Geometry: final body of the model. Coordinates: model frame, mm. A direction names the side the tool comes from. Give positions to 0.01 mm unless a question says otherwise; leave off trailing zeros. Order: outer loops, then holes, each group sorted by start corner. A loop starts at its lowest first (then second) coordinate and runs counter-clockwise, first axis right, second up. Notation, with made-up numbers: (-8.75, 43.5) - (40.25, 43.5) arc R6 ccw to (40.25, 47.5) - close; hole circle Ø11 at (-13.5, -34.5). An arc over 180 degrees is marked (long way). Use one line per item in the form item = value.
from build123d import *

# Parameters (mm, degrees)
EXTRUDE_1_DEPTH     = 20
SKETCH_2_R          = 3
CUT_EXTRUDE_1_DEPTH = 42.952353927
SKETCH_3_R          = 3
CUT_EXTRUDE_2_DEPTH = 42.952353927
SKETCH_4_W          = 2
SKETCH_4_H          = 6
EXTRUDE_1_2_DEPTH   = 1.5
SKETCH_5_W          = 4
SKETCH_5_H          = 6
CUT_EXTRUDE_3_DEPTH = 1.5
SKETCH_6_W          = 6
SKETCH_6_H          = 2
EXTRUDE_2_DEPTH     = 1.5
SKETCH_7_W          = 6
SKETCH_7_H          = 4
CUT_EXTRUDE_4_DEPTH = 1.5
SKETCH_8_W          = 6
SKETCH_8_H          = 2
EXTRUDE_3_DEPTH     = 1.5
SKETCH_10_W         = 6
SKETCH_10_H         = 2
CUT_EXTRUDE_6_DEPTH = 1.5
SKETCH_11_W         = 2
SKETCH_11_H         = 6
EXTRUDE_4_DEPTH     = 1.5
SKETCH_12_W         = 2
SKETCH_12_H         = 6
CUT_EXTRUDE_7_DEPTH = 1.5
RIB_1_DEPTH         = 2.6
RIB_START           = -2.6
RIB_2_DEPTH         = 2.6


# Read off the part's stored shape, not the designer's step: 筋1, 筋2
with BuildPart() as part:
    # 草图1 → Extrude 1 (new body)
    with BuildSketch(Plane.XY):
        Polygon((28, 0), (0, 0), (0, 28), (4, 28), (4, 4), (28, 4), align=None)
    extrude(amount=EXTRUDE_1_DEPTH)

    # 草图2 → 切除-拉伸1 (cut, through all)
    with BuildSketch(Plane(origin=(0, 4, 0), x_dir=(1, 0, 0), z_dir=(0, 1, 0))):
        with Locations(Location((17, -10, 0), (0, 0, 180))):
            Circle(SKETCH_2_R)
    extrude(amount=-CUT_EXTRUDE_1_DEPTH, mode=Mode.SUBTRACT)

    # 草图3 → 切除-拉伸2 (cut, through all)
    with BuildSketch(Plane(origin=(4, 0, 0), x_dir=(0, 0, -1), z_dir=(1, 0, 0))):
        with Locations((-10, 17)):
            Circle(SKETCH_3_R)
    extrude(amount=-CUT_EXTRUDE_2_DEPTH, mode=Mode.SUBTRACT)

    # 草图4 → Extrude 1 2 (add)
    with BuildSketch(Plane.XZ):
        with Locations((3, 10)):
            Rectangle(SKETCH_4_W, SKETCH_4_H)
    extrude(amount=EXTRUDE_1_2_DEPTH)

    # 草图5 → 切除-拉伸3 (cut)
    with BuildSketch(Plane.XZ):
        with Locations((6, 10)):
            Rectangle(SKETCH_5_W, SKETCH_5_H)
    extrude(amount=-CUT_EXTRUDE_3_DEPTH, mode=Mode.SUBTRACT)

    # 草图6 → 凸台-拉伸2 (add)
    with BuildSketch(Plane.ZY):
        with Locations((10, 3)):
            Rectangle(SKETCH_6_W, SKETCH_6_H)
    extrude(amount=EXTRUDE_2_DEPTH)

    # 草图7 → 切除-拉伸4 (cut)
    with BuildSketch(Plane.ZY):
        with Locations((10, 6)):
            Rectangle(SKETCH_7_W, SKETCH_7_H)
    extrude(amount=-CUT_EXTRUDE_4_DEPTH, mode=Mode.SUBTRACT)

    # 草图8 → 凸台-拉伸3 (add)
    with BuildSketch(Plane.ZY):
        with Locations((10, 25)):
            Rectangle(SKETCH_8_W, SKETCH_8_H)
    extrude(amount=EXTRUDE_3_DEPTH)

    # 草图10 → 切除-拉伸6 (cut)
    with BuildSketch(Plane.ZY):
        with Locations((10, 23)):
            Rectangle(SKETCH_10_W, SKETCH_10_H)
    extrude(amount=-CUT_EXTRUDE_6_DEPTH, mode=Mode.SUBTRACT)

    # 草图11 → 凸台-拉伸4 (add)
    with BuildSketch(Plane.XZ):
        with Locations((25, 10)):
            Rectangle(SKETCH_11_W, SKETCH_11_H)
    extrude(amount=EXTRUDE_4_DEPTH)

    # 草图12 → 切除-拉伸7 (cut)
    with BuildSketch(Plane.XZ):
        with Locations((23, 10)):
            Rectangle(SKETCH_12_W, SKETCH_12_H)
    extrude(amount=-CUT_EXTRUDE_7_DEPTH, mode=Mode.SUBTRACT)

    # 筋1 outline → 筋1 (add)
    with BuildSketch(Plane.XY):
        Polygon((6, 23), (6, 28), (4, 28), (4, 4), (28, 4), (28, 6), (23, 6), align=None)
    extrude(amount=RIB_1_DEPTH)

    # 筋2 outline → 筋2 (add)
    with BuildSketch(Plane.XY.offset(20).offset(RIB_START)):
        Polygon((6, 23), (6, 28), (4, 28), (4, 4), (28, 4), (28, 6), (23, 6), align=None)
    extrude(amount=RIB_2_DEPTH)


solid = part.part
(1) Pull-direction query (X, two-part tool) for faces 1 (the face through (26, -1, 10)), 2 (the face through (6, 1.5, 10)), 3 (the face through (2, -1, 10)), 4 (the face through (1, 6, 13)); classes: released by +X, released by -X, zero draft, split by the parting line, or undercut.
Computed values:
face_1 = released by +X
face_2 = undercut
face_3 = released by -X
face_4 = zero draft
(2) Cut plane A-A on x = 17. Output: boundary loops of the cut face in (y, z), plus the area to 3 significant figures.
Computed values:
outline = (0, 0) - (12, 0) - (12, 2.6) - (4, 2.6) - (4, 7) - (0, 7) - close; (0, 13) - (4, 13) - (4, 17.4) - (12, 17.4) - (12, 20) - (0, 20) - close
area = 97.6 mm²
(3) Ray query, line 1 along Y through (x, z) = (0.8, 10); line 2 along Z through (x, y) = (17, 2.9); line 3 along X through (y, z) = (0.5, 11.25). Return the intervals inside material, ascending.
Computed values:
line_1 = 0 to 4, 8 to 14, 20 to 22, 24 to 28
line_2 = 0 to 7, 13 to 20
line_3 = 0 to 4, 8 to 14.27, 19.73 to 22, 24 to 28
(4) Reachability of faces 5 (the face through (-1, 3, 7)), 6 (the face through (6, 25, 19)), 7 (the face through (25, -1, 13)), 8 (the face through (1, 6, 7)), 9 (the face through (-1, 2, 10)) from +Z, -Z, +X, -X, +Y, -Y: full face, straight path, thin tool, end or side. Return the list, or none.
Computed values:
face_5 = -Z, -X, +Y, -Y
face_6 = +Z, -Z, +X, +Y
face_7 = +Z, +X, -X, -Y
face_8 = -X
face_9 = +Z, -Z, -X, -Y
(5) Cut plane C-C on z = 5.25. Output: boundary loops of the cut face in (x, y), plus the area to 3 significant figures.
Computed values:
outline = (0, 0) - (28, 0) - (28, 4) - (4, 4) - (4, 28) - (0, 28) - close
area = 208 mm²
(6) Contact query for flat-ended pins moving along their axis: pin 1 Ø12 at (y, z) = (13.5, 5) entering from -X; pin 2 Ø10 at (x, z) = (14.5, 4.5) entering from -Y; pin 3 Ø0.8 at (x, y) = (3.5, -1) entering from +Z; pin 4 Ø5 at (x, z) = (17, 10) entering from -Y. Output: stop coordinate, or through.
Computed values:
pin_1 = 0
pin_2 = 0
pin_3 = 13
pin_4 = through
(7) Cut plane D-D on x = 21.5. Output: boundary loops of the cut face in (y, z), plus the area to 3 significant figures.
Computed values:
outline = (0, 0) - (7.5, 0) - (7.5, 2.6) - (4, 2.6) - (4, 17.4) - (7.5, 17.4) - (7.5, 20) - (0, 20) - close
area = 98.2 mm²
